Can you work these out from the model? Positions are in its coordinate system, mm. A direction names the side the tool comes from. Coordinates: 2 decimals unless noted, no trailing zeros. Order: outer loops, then holes, each group sorted by start corner. A loop starts at its lowest first (then second) coordinate and runs counter-clockwise, first axis right, second up. Notation, with made-up numbers: (51, 38) -> (78, 38) arc R30 cw to (78, 61) -> close; hole circle Ø6 at (79, 71). An arc over 180 degrees is marked (long way). Answer in a Markdown table with one row per item.
```python
from build123d import *

# Parameters (mm, degrees)
BOSS_EXTRUDE1_DEPTH = 23
CUT_EXTRUDE1_START  = 24
CUT_EXTRUDE1_DEPTH  = 12
SKETCH5_R           = 6
CUT_EXTRUDE2_DEPTH  = 76.822160349
SKETCH6_R           = 17
CUT_EXTRUDE3_DEPTH  = 46
SKETCH10_R          = 4
CUT_EXTRUDE6_DEPTH  = 20
SKETCH11_R          = 3
CUT_EXTRUDE7_DEPTH  = 63.681735814


# Read off the part's stored shape, not the designer's step: Cut-Extrude1
with BuildPart() as part:
    # Sketch1 → Boss-Extrude1 (new, symmetric)
    with BuildSketch(Plane.XY):
        with BuildLine():
            Line((-22.627416998, 8), (-28, 8))
            Line((-28, 8), (-28, 24))
            Line((-28, 24), (-54, 24))
            Line((-54, 24), (-54, 36))
            Line((-54, 36), (-31.749015733, 36))
            ThreePointArc((-31.749015733, 36), (0, 48), (31.749015733, 36))
            Line((31.749015733, 36), (54, 36))
            Line((54, 36), (54, 24))
            Line((54, 24), (28, 24))
            Line((28, 24), (28, 8))
            Line((28, 8), (22.627416998, 8))
            ThreePointArc((22.627416998, 8), (0, 24), (-22.627416998, 8))
        make_face()
    extrude(amount=BOSS_EXTRUDE1_DEPTH, both=True)

    # Cut-Extrude1 outline → Cut-Extrude1 (cut)
    with BuildSketch(Plane(origin=(0, 0, 0), x_dir=(1, 0, 0), z_dir=(0, 1, 0)).offset(CUT_EXTRUDE1_START)):
        with BuildLine():
            Line((-54, -23), (-48.856934001, -23))
            ThreePointArc((-48.856934001, -23), (-52.698550436, -11.784005345), (-54, 0))
            Line((-54, 0), (-54, -23))
        make_face()
        with BuildLine():
            Line((-54, 23), (-54, 0))
            ThreePointArc((-54, 0), (-52.698550436, 11.784005345), (-48.856934001, 23))
            Line((-48.856934001, 23), (-54, 23))
        make_face()
        with BuildLine():
            ThreePointArc((54, 0), (52.698550436, -11.784005345), (48.856934001, -23))
            Line((48.856934001, -23), (54, -23))
            Line((54, -23), (54, 0))
        make_face()
        with BuildLine():
            ThreePointArc((48.856934001, 23), (52.698550436, 11.784005345), (54, 0))
            Line((54, 0), (54, 23))
            Line((54, 23), (48.856934001, 23))
        make_face()
    extrude(amount=CUT_EXTRUDE1_DEPTH, mode=Mode.SUBTRACT)

    # Sketch5 → Cut-Extrude2 (cut, through all)
    with BuildSketch(Plane(origin=(0, 0, 0), x_dir=(1, 0, 0), z_dir=(0, 1, 0))):
        with Locations(Location((-39, 0, 0), (0, 0, 90))):
            Circle(SKETCH5_R)
        with Locations(Location((39, 0, 0), (0, 0, 90))):
            Circle(SKETCH5_R)
    extrude(amount=CUT_EXTRUDE2_DEPTH, mode=Mode.SUBTRACT)

    # Sketch6 → Cut-Extrude3 (cut)
    with BuildSketch(Plane(origin=(0, 36, 0), x_dir=(1, 0, 0), z_dir=(0, 1, 0))):
        with Locations((-39, 0)):
            Circle(SKETCH6_R)
        with Locations((39, 0)):
            Circle(SKETCH6_R)
    extrude(amount=CUT_EXTRUDE3_DEPTH, mode=Mode.SUBTRACT)

    # Sketch10 → Cut-Extrude6 (cut)
    with BuildSketch(Plane(origin=(0, 50, 0), x_dir=(1, 0, 0), z_dir=(0, 1, 0))):
        with Locations(Location((0, 0, 0), (0, 0, 270))):
            Circle(SKETCH10_R)
    extrude(amount=-CUT_EXTRUDE6_DEPTH, mode=Mode.SUBTRACT)

    # Sketch11 → Cut-Extrude7 (cut, through all)
    with BuildSketch(Plane(origin=(0, 30, 0), x_dir=(1, 0, 0), z_dir=(0, 1, 0))):
        with Locations(Location((0, 0, 0), (0, 0, 270))):
            Circle(SKETCH11_R)
    extrude(amount=-CUT_EXTRUDE7_DEPTH, mode=Mode.SUBTRACT)


solid = part.part
```
(1) On a 3-axis mill with a long thin cutter (end or side, diameter ignored), from which of +Z, -Z, +X, -X, +Y, -Y can I reach the whole of each face in a straight line? I mean faces 1 (the cylindrical face through (-22, 39, 0)), 2 (the flat face through (-28, 16, 0)), 3 (the flat face through (3, 30, 1)), 4 (the flat face through (34, 36, 5)). Say none if no direction works.
Response values:
| item | result |
|---|---|
| face 1 | -X, +Y |
| face 2 | +Z, -Z, -X, -Y |
| face 3 | +Y |
| face 4 | +X, +Y |
(2) Suppose I cut it at D-D (x = 0). Please give me the cut outline in (y, z), and give its area (3 significant figures).
Response values:
| item | result |
|---|---|
| outline | (24, -23) -> (48, -23) -> (48, -4) -> (30, -4) -> (30, -3) -> (24, -3) -> close; (24, 3) -> (30, 3) -> (30, 4) -> (48, 4) -> (48, 23) -> (24, 23) -> close |
| area | 924 mm2 |
(3) Suppose I cut it at C-C (y = 14.5). Please give me the cut outline in (x, z).
Response values:
| item | result |
|---|---|
| outline | (-28, -23) -> (-19.12, -23) -> (-19.12, 23) -> (-28, 23) -> close; (19.12, -23) -> (28, -23) -> (28, 23) -> (19.12, 23) -> close |
(4) Suppose I cut it at B-B (y = 26). Please give me the cut outline in (x, z), and give its area (3 significant figures).
Response values:
| item | result |
|---|---|
| outline | (-48.86, -23) -> (48.86, -23) arc R54 ccw to (48.86, 23) -> (-48.86, 23) arc R54 ccw to start; hole circle Ø12 at (-39, 0); hole circle Ø6 at (0, 0); hole circle Ø12 at (39, 0) |
| area | 4,560 mm2 |
(5) Will these pins go through, and if not, where does the flat tip stop? pin 1 Ø13 at (x, z) = (37, 8) entering from -Y; pin 2 Ø7 at (x, z) = (-39, 0) entering from +Y; pin 3 Ø6 at (x, z) = (10, 13) entering from +Y; pin 4 Ø1.5 at (x, z) = (-12, 14) entering from -Y.
Response values:
| item | result |
|---|---|
| pin 1 | y = 24 |
| pin 2 | through |
| pin 3 | y = 47.49 |
| pin 4 | y = 20.33 |
(6) Suppose I cut it at A-A (x = 39). Please give me the cut outline in (y, z), and give its area (3 significant figures).
Response values:
| item | result |
|---|---|
| outline | (24, -23) -> (36, -23) -> (36, -6) -> (24, -6) -> close; (24, 6) -> (36, 6) -> (36, 23) -> (24, 23) -> close |
| area | 408 mm2 |
(7) I need wall thicknesses on line 1 (Z direction, x = 0, y = 37); line 2 (Z direction, x = 0, y = 28); line 3 (X direction, y = 41.5, z = 0). Which ranges of each line are inside material? Lowest first, please. Write a range as [from, to].
Response values:
| item | result |
|---|---|
| line 1 | [-23, -4], [4, 23] |
| line 2 | [-23, -3], [3, 23] |
| line 3 | [-22, -4], [4, 22] |
